CAD build for the part. Positions are in the model's coordinates, mm. A direction names the side the tool comes from. Round coordinates to 2 decimals unless told otherwise and drop trailing zeros. Loops run counter-clockwise (first coordinate to the right, second up) from the corner with the lowest first, then second, coordinate; pieces in that order, holes last. Notation, with made-up numbers: (13, 12) - (61, 12) arc R17 cw to (61, 43) - close; hole circle Ø9 at (71, -26). An arc over 180 degrees is marked (long way). One line per question, with ' | ' between items.
```python
from build123d import *

# Parameters (mm, degrees)
BOSS_EXTRUDE1_DEPTH = 129.54
SKETCH2_R           = 2.54
CUT_EXTRUDE1_DEPTH  = 2.54
SKETCH4_R           = 2.54
CUT_EXTRUDE2_DEPTH  = 2.54
CUT_EXTRUDE3_DEPTH  = 130.5400001
SHELL1_T            = -2.54


with BuildPart() as part:
    # Sketch1 → Boss-Extrude1 (new body)
    with BuildSketch(Plane.XY):
        with BuildLine():
            Line((127, 0), (0, 0))
            Line((0, 0), (-127, 0))
            ThreePointArc((-127, 0), (0, 127), (127, 0))
        make_face()
    extrude(amount=BOSS_EXTRUDE1_DEPTH)

    # Sketch2 → Cut-Extrude1 (cut)
    with BuildSketch(Plane(origin=(0, 127, 129.54), x_dir=(1, 0, 0), z_dir=(0, 1, 0))):
        with Locations((0, 29.845)):
            Circle(SKETCH2_R)
        with Locations((0, 99.695)):
            Circle(SKETCH2_R)
    extrude(amount=-CUT_EXTRUDE1_DEPTH, mode=Mode.SUBTRACT)

    # Sketch4 → Cut-Extrude2 (cut)
    with BuildSketch(Plane(origin=(53.676536994, 115.099215359, 129.54), x_dir=(0.906293034, -0.422649898, 0), z_dir=(0.422649898, 0.906293034, 0))):
        with Locations((0, 29.845)):
            Circle(SKETCH4_R)
        with Locations((0, 99.695)):
            Circle(SKETCH4_R)
    extrude(amount=-CUT_EXTRUDE2_DEPTH, mode=Mode.SUBTRACT)

    # Sketch5 → Cut-Extrude3 (cut, through all)
    with BuildSketch(Plane.XY.offset(129.54)):
        with BuildLine():
            Line((72.844207417, 104.032309625), (0, 0))
            Line((0, 0), (127, 0))
            ThreePointArc((127, 0), (112.650375814, 58.642073881), (72.844207417, 104.032309625))
        make_face()
    extrude(amount=-CUT_EXTRUDE3_DEPTH, mode=Mode.SUBTRACT)

    # Shell1
    shell1_openings = [part.faces().sort_by_distance(p)[0] for p in [
        (-63.5, 0, 64.77),
        (36.422103708, 52.016154812, 64.77),
    ]]
    offset(amount=SHELL1_T, openings=shell1_openings, kind=Kind.INTERSECTION)


solid = part.part
```
(1) Cut at C-C, the plane z = 9. Write the cut outline in (x, y).
Results found:
outline: (-127, 0) - (-124.46, 0) arc R124.46 cw to (71.39, 101.95) - (72.84, 104.03) arc R127 ccw to start
(2) Cut at B-B, the plane x = -40.5. Write the cut outline in (y, z).
Results found:
outline: (0, 0) - (120.37, 0) - (120.37, 129.54) - (0, 129.54) - (0, 127) - (117.69, 127) - (117.69, 2.54) - (0, 2.54) - close
(3) Drop flat-ended pins along their axis: P1, Ø1.5, axis at x = 5, z = 88, coming from the -Y side; P2, Ø2, axis at x = -73.5, z = 82.5, coming from the -Y side; P3, Ø8, axis at x = -5.5, z = 55.5, coming from the +Y side. Give the stop position or say it passes through.
Results found:
P1: stops at y = 124.33 | P2: stops at y = 99.7 | P3: stops at y = 126.99
(4) Cut at A-A, the plane y = 14.5. Write the cut outline in (x, z).
Results found:
outline: (-126.17, 0) - (10.15, 0) - (10.15, 2.54) - (-123.61, 2.54) - (-123.61, 127) - (10.15, 127) - (10.15, 129.54) - (-126.17, 129.54) - close
(5) Probe L1, parallel to Z at x = 0, y = 125.1 (3 decimals); L2, parallel to Z at x = -53, y = 11; L3, parallel to X at y = 109, z = 76. List the from-to ranges inside material, lowest first.
Results found:
L1: z = 0 to 27.305, 32.385 to 97.155, 102.235 to 129.54 | L2: z = 0 to 2.54, 127 to 129.54 | L3: x = -65.18 to -60.08, 60.08 to 65.18
(6) Tool access for faces 1 (the face through (71.665, 102.349, 93.859)), 2 (the face through (-1.101, 123.208, 104.654)), 3 (the face through (52.6, 112.8, 99.7)), 4 (the face through (-26, 64, 0)), 5 (the face through (-0.331, 125.748, 27.327)): list every direction of +Z, -Z, +X, -X, +Y, -Y with a clear straight run to the whole face (end or side of a thin tool).
Results found:
face 1: +Z, -Z, +X, -Y | face 2: -Y | face 3: none | face 4: -Z, +X, -X, +Y, -Y | face 5: +Y
(7) Two-plate mould, pull along X, no slides. Class faces 6 (the face through (50.85, 115.04, 29.73)), 7 (the face through (51.465, 110.525, 99.624)), 8 (the face through (-26, 64, 129.54)), 9 (the face through (-60.36, 111.74, 63.86)): released by +X, released by -X, zero draft, split by the parting line, or undercut.
Results found:
face 6: undercut | face 7: undercut | face 8: zero draft | face 9: split by the parting line
